Autodesk Inventor part; units mm, degrees
ref_plane "Work Plane1" through (165, 1216, -85) normal (0, 0.8011494, -0.5984644) x (1, 0, 0)
ref_plane "YZ Plane" through (0, 0, 0) normal (1, 0, 0) x (0, 1, 0)
ref_plane "XZ Plane" through (0, 0, 0) normal (0, 1, 0) x (-1, 0, 0)
sketch "Sketch1" plane through (0, 0, 0) normal (0, 1, 0) x (-1, 0, 0)
  line L0 (165, 215) -> (-165, 215)
  line L1 (-165, 215) -> (-165, -215)
  line L2 (-165, -215) -> (165, -215)
  line L3 (165, -215) -> (165, 215)
  line L4 (165, 215) -> (-165, -215) construction
  line L5 (-165, 215) -> (165, -215) construction
  point P0 (0, 0)
  dimension "d0" = 330
  dimension "d1" = 430
extrude "Extrusion1" add sketch "Sketch1" along normal blind 816
move faces "Move1" translate (0, 400, 0) faces at (55, 816, 71.6667)
chamfer "Chamfer1" distance 300 angle 53.24 1 edges at (0, 1216, 215) measured on face at (55, 1216, 71.6667)
chamfer "Chamfer2" distance 130 angle 36.76 1 edges at (0, 1216, -215) measured on face at (55, 1216, -171.6667)
ref_plane "Work Plane1" through (165, 1216, -85) normal (0, 0.8011494, -0.5984644) x (1, 0, 0)
sketch "Sketch2" plane through (165, 1216, -85) normal (0, 0.8011494, -0.5984644) x (1, 0, 0)
  line L0 (-330, 0) -> (0, 0)
  line L1 (-330, 487.3879) -> (-330, 0)
  line L2 (0, 0) -> (-330, 0)
  line L3 (-330, 0) -> (-330, 430)
  line L4 (-330, 430) -> (0, 430)
  line L5 (0, 430) -> (0, 0)
  point P0 (-165, 659.6351)
extrude "Extrusion2" add sketch "Sketch2" against normal blind 358.4
sketch "Sketch3" plane through (-165, 1216, -85) normal (0, 0.8011494, -0.5984644) x (1, 0, 0)
  circle A0 centre (165, 180) radius 80
  point P0 (165, 659.6351)
extrude "Extrusion3" cut sketch "Sketch3" against normal blind 400
sketch "Sketch4" plane through (0, 0, 0) normal (0, -1, 0) x (1, 0, 0)
  line L0 (165, 215) -> (-165, 215)
  line L1 (-165, 215) -> (-165, -215)
  line L2 (-165, -215) -> (165, -215)
  line L3 (165, -215) -> (165, 215)
  line L4 (165, 215) -> (-165, -215) construction
  line L5 (-165, 215) -> (165, -215) construction
  point P0 (0, 0)
extrude "Extrusion4" cut sketch "Sketch4" against normal blind 10
sketch "Sketch5" plane through (0, 10, 0) normal (0, -1, 0) x (1, 0, 0)
  line L0 (205, 255) -> (-205, 255)
  line L1 (-205, 255) -> (-205, -255)
  line L2 (-205, -255) -> (205, -255)
  line L3 (205, -255) -> (205, 255)
  line L4 (205, 255) -> (-205, -255) construction
  line L5 (-205, 255) -> (205, -255) construction
  point P0 (0, 0)
extrude "Extrusion5" add sketch "Sketch5" along normal blind 10
properties part number "MountBase"
Here's how the part is built. I have some questions about the finished solid (model axes, mm). A direction names the side the tool comes from. Coordinates: 2 decimals unless noted, no trailing zeros. Order: outer loops, then holes, each group sorted by start corner. A loop starts at its lowest first (then second) coordinate and runs counter-clockwise, first axis right, second up.
1) I need wall thicknesses on line 1 (Z direction, x = -47.5, y = 174.5); line 2 (Y direction, x = 30, z = -150); line 3 (Y direction, x = -176, z = -3). Which ranges of each line are inside material? Lowest first, please.
2) We'd pull the mould along Z, two halves only. Please class faces 1 (the face through (-1.12, 787.145, 9.283)), 2 (the face through (165, 568, -9)), 3 (the face through (73.9, 968.63, -86.64)), 4 (the face through (-2, 407, 215)): +Z half, -Z half, draft (parallel to the pull), parting line (faces both ways), or undercut.
3) Will these pins go through, and if not, where does the flat tip stop? pin 1 (12 mm diameter, centred on x = 95.5, y = 993, fed in from +Z); pin 2 (4 mm diameter, centred on y = 978.5, z = -26, fed in from +X); pin 3 (1 mm diameter, centred on x = 127, y = 577, fed in from -Z).
4) Which directions (+Z, -Z, +X, -X, +Y, -Y) give clear straight access to the entire face, cutting with the end or side of a thin tool? Please do faces 5 (the face through (-3, 0, 4)), 6 (the face through (2, 336, -215)), 7 (the face through (-165, 568, -9)), 8 (the face through (-185, 10, 4)).
5) Imagine slicing it at B-B on y = 211.5. List the corners of the cut face in (x, z) for me, and give its area (3 significant figures).
6) Imagine slicing it at C-C on z = 128.5. List the corners of the cut face in (x, y) for me.
Response values:
1. line 1: z = -215 to 215
1. line 2: y = 0 to 878.32, 1126.16 to 1167.44
1. line 3: y = 0 to 10
2. face 1: undercut
2. face 2: draft
2. face 3: undercut
2. face 4: +Z half
3. pin 1: stops at z = 86.06
3. pin 2: stops at x = 165
3. pin 3: stops at z = -215
4. face 5: +Z, -Z, +X, -X, -Y
4. face 6: -Z, +X, -X
4. face 7: +Z, -Z, -X, +Y
4. face 8: none
5. outline: (-165, -215) - (165, -215) - (165, 215) - (-165, 215) - close
5. area: 142,000 mm2
6. outline: (-205, 0) - (205, 0) - (205, 10) - (165, 10) - (165, 930.19) - (-165, 930.19) - (-165, 10) - (-205, 10) - close
